Geometry check sheet. Reference: the model listing, model coordinates, mm. A direction names the side the tool comes from. Coordinates: 2 decimals unless noted, no trailing zeros. Order: outer loops, then holes, each group sorted by start corner. A loop starts at its lowest first (then second) coordinate and runs counter-clockwise, first axis right, second up. Notation, with made-up numbers: M 55,71 L 98,71 A19 ccw 98,101 Z; hole C 76,24.5 d2. An arc over 180 degrees is marked long. One line per item, written item: value. Start each with the question number.
1) Thickness scan on L1, parallel to Y at x = -18.5, z = 0.75; L2, parallel to Y at x = -54, z = 1.15; L3, parallel to Y at x = -28.5, z = 0.75. Record the ranges inside material, lowest first. Write a range as from..to.
2) Sectioned sample at A-A, the plane x = -54. Enter the section's corners in (y, z).
3) Sectioned sample at B-B, the plane z = 0.5. Enter the section's corners in (x, y), then the cut area to 3 significant figures.
4) Go/stop test with flat-tipped pins: P1, Ø5, axis at x = -73.5, y = 23.5, coming from the -Z side; P2, Ø3.5, axis at x = -102, y = 28, coming from the +Z side. Record where each tip stops, or that it passes through.
5) Access from +Z, -Z, +X, -X, +Y, -Y to the whole of each face (thin tool, end or side, straight path). Record for faces 1 (the flat face through (-98, 24, 1.5)), 2 (the flat face through (-78, 69, 1)), 3 (the flat face through (-34, 47, 2)).
6) Sectioned sample at C-C, the plane x = -17. Enter the section's corners in (y, z).
7) Draft check along X on faces 4 (the flat face through (0, 34, 1)), 5 (the flat face through (-78, 35, 0)), 6 (the cylindrical face through (-107.994, 25.764, 2.26)). Enter one of: pulls with the +X half, pulls with the -X half, needs draft (parallel to the pull), parting line crosses it, or undercut.
8) Sectioned sample at D-D, the plane y = 47. Enter the section's corners in (x, z).
```python
from build123d import *

# Parameters (mm, degrees)
IZIM1_W                     = 153
IZIM1_H                     = 69
Y_KSEKLIK_EKSTR_ZYON1_DEPTH = 3
IZIM2_R                     = 3
IZIM2_R_2                   = 4
IZIM2_R_3                   = 6
IZIM2_W                     = 19
IZIM2_H                     = 13
KES_EKSTR_ZYON1_DEPTH       = 3
IZIM4_R                     = 5.5
IZIM4_R_2                   = 6
KES_EKSTR_ZYON2_DEPTH       = 1.5
IZIM5_W                     = 13
IZIM5_H                     = 10
KES_EKSTR_ZYON4_DEPTH       = 1.5
IZIM7_W                     = 10
IZIM7_H                     = 6.5
KES_EKSTR_ZYON5_DEPTH       = 1.5
RADYUS1_R                   = 2


with BuildPart() as part:
    # Çizim1 → Yükseklik-Ekstrüzyon1 (new body)
    with BuildSketch(Plane.XY):
        with Locations((-76.5, 34.5)):
            Rectangle(IZIM1_W, IZIM1_H)
    extrude(amount=Y_KSEKLIK_EKSTR_ZYON1_DEPTH)

    # Çizim2 → Kes-Ekstrüzyon1 (cut)
    with BuildSketch(Plane.XY.offset(3)):
        with Locations((-133.25, 25)):
            Circle(IZIM2_R)
        with Locations((-102, 25.5)):
            Circle(IZIM2_R_2)
        with Locations((-33.75, 25)):
            Circle(IZIM2_R)
        with Locations((-54, 49)):
            Circle(IZIM2_R_3)
        with Locations((-24.5, 47.5)):
            Rectangle(IZIM2_W, IZIM2_H)
    extrude(amount=-KES_EKSTR_ZYON1_DEPTH, mode=Mode.SUBTRACT)

    # Çizim4 → Kes-Ekstrüzyon2 (cut)
    with BuildSketch(Plane.XY.offset(3)):
        with Locations((-133.25, 25)):
            Circle(IZIM4_R)
        with Locations((-102, 25.5)):
            Circle(IZIM4_R_2)
        with Locations((-33.75, 25)):
            Circle(IZIM4_R_2)
    extrude(amount=-KES_EKSTR_ZYON2_DEPTH, mode=Mode.SUBTRACT)

    # Çizim5 → Kes-Ekstrüzyon4 (cut)
    with BuildSketch(Plane.XY.offset(3)):
        with Locations((-15.75, 29.1)):
            Rectangle(IZIM5_W, IZIM5_H)
    extrude(amount=-KES_EKSTR_ZYON4_DEPTH, mode=Mode.SUBTRACT)

    # Çizim7 → Kes-Ekstrüzyon5 (cut)
    with BuildSketch(Plane.XY.offset(1.5)):
        with Locations((-15.75, 28.85)):
            Rectangle(IZIM7_W, IZIM7_H)
    extrude(amount=-KES_EKSTR_ZYON5_DEPTH, mode=Mode.SUBTRACT)

    # Radyus1
    radyus1_edges = [part.edges().sort_by_distance(p)[0] for p in [
        (-22.25, 24.1, 2.25),
        (-22.25, 34.1, 2.25),
        (-9.25, 34.1, 2.25),
        (-9.25, 24.1, 2.25),
    ]]
    fillet(radyus1_edges, radius=RADYUS1_R)


solid = part.part
```
Final values:
1. L1: y = 0..25.6, 32.1..41, 54..69
1. L2: y = 0..43, 55..69
1. L3: y = 0..41, 54..69
2. outline: M 0,0 L 43,0 L 43,3 L 0,3 Z; M 55,0 L 69,0 L 69,3 L 55,3 Z
3. outline: M -153,0 L 0,0 L 0,69 L -153,69 Z; hole C -133.25,25 d6; hole C -102,25.5 d8; hole C -54,49 d12; hole C -33.75,25 d6; hole M -34,41 L -15,41 L -15,54 L -34,54 Z; hole M -20.75,25.6 L -10.75,25.6 L -10.75,32.1 L -20.75,32.1 Z
3. area: 10,000 mm^2
4. P1: stops at z = 0
4. P2: stops at z = 1.5
5. face 1: +Z
5. face 2: +Z, -Z, +X, -X, +Y
5. face 3: +Z, -Z
6. outline: M 0,0 L 25.6,0 L 25.6,1.5 L 24.1,1.5 L 24.1,3 L 0,3 Z; M 32.1,0 L 41,0 L 41,3 L 34.1,3 L 34.1,1.5 L 32.1,1.5 Z; M 54,0 L 69,0 L 69,3 L 54,3 Z
7. face 4: pulls with the +X half
7. face 5: needs draft
7. face 6: undercut
8. outline: M -153,0 L -59.66,0 L -59.66,3 L -153,3 Z; M -48.34,0 L -34,0 L -34,3 L -48.34,3 Z; M -15,0 L 0,0 L 0,3 L -15,3 Z
